```python
from build123d import *

# Parameters (mm, degrees)
F1_DEPTH = 12.7
F2_R     = 3.302
F3_DEPTH = 41.5002601562
F4_W     = 102.0685225816
F4_H     = 3.4845213629
F5_DEPTH = 25
F6_R     = 2


# Not quite as in the source:
# - ends of sketch curves that miss each other by under 0.0002 mm in the source are joined
# - the dataset's text gives a spline's control points without its knots; the knots are read off the source's solid


with BuildPart() as f1:
    # F0 (on Front) → F1 (new body)
    with BuildSketch(Plane.XZ):
        with BuildLine():
            Line((-8, 0), (0, 0))
            add(Edge.make_bspline(
                [(0, 0), (0, 16.0348825157), (7.430841215, 33.6514413357), (23.5, 33.5)],
                knots=[0, 0, 0, 0, 40.9206549312, 40.9206549312, 40.9206549312, 40.9206549312], degree=3))
            add(Edge.make_bspline(
                [(47, 0), (47, 16.0348825157), (39.569158785, 33.6514413357), (23.5, 33.5)],
                knots=[0, 0, 0, 0, 40.9206549312, 40.9206549312, 40.9206549312, 40.9206549312], degree=3))
            Line((47, 0), (55, 0))
            add(Edge.make_bspline(
                [(55, 0), (55, 2.3133051501), (54.8084752548, 5.6604865088), (54.3346414744, 8.9941225704), (54.1644875118, 10.0000161913)],
                knots=[0, 0, 0, 0, 0.125, 0.1792883855, 0.1792883855, 0.1792883855, 0.1792883855], degree=3))
            add(Edge.make_bspline(
                [(54.1644875118, 10.0000161913), (53.9428588652, 11.3102110198), (53.2041802455, 14.9199242801), (51.403557473, 20.6965522199), (48.312647429, 27.0635606249), (44.7757382973, 31.8590791464), (41.27501086, 35.2044913237), (38.3020149436, 37.39930019), (34.9881581098, 39.2038242784), (31.3670929719, 40.5407901401), (27.6491274865, 41.3170292606), (25.11417344, 41.4919330376), (23.9092731988, 41.5002601562)],
                knots=[0.1792883855, 0.1792883855, 0.1792883855, 0.1792883855, 0.25, 0.375, 0.5, 0.625, 0.6875, 0.75, 0.8125, 0.875, 0.9375, 0.9926226885, 0.9926226885, 0.9926226885, 0.9926226885], degree=3))
            Line((23.9092731988, 41.5002601562), (23.5, 41.5002601562))
            Line((23.5, 41.5002601562), (23.0907268012, 41.5002601562))
            add(Edge.make_bspline(
                [(-7.1644875118, 10.0000161913), (-6.9428588652, 11.3102110198), (-6.2041802455, 14.9199242801), (-4.403557473, 20.6965522199), (-1.312647429, 27.0635606249), (2.2242617027, 31.8590791464), (5.72498914, 35.2044913237), (8.6979850564, 37.39930019), (12.0118418902, 39.2038242784), (15.6329070281, 40.5407901401), (19.3508725135, 41.3170292606), (21.88582656, 41.4919330376), (23.0907268012, 41.5002601562)],
                knots=[0.1792883855, 0.1792883855, 0.1792883855, 0.1792883855, 0.25, 0.375, 0.5, 0.625, 0.6875, 0.75, 0.8125, 0.875, 0.9375, 0.9926226885, 0.9926226885, 0.9926226885, 0.9926226885], degree=3))
            add(Edge.make_bspline(
                [(-8, 0), (-8, 2.3133051501), (-7.8084752548, 5.6604865088), (-7.3346414744, 8.9941225704), (-7.1644875118, 10.0000161913)],
                knots=[0, 0, 0, 0, 0.125, 0.1792883855, 0.1792883855, 0.1792883855, 0.1792883855], degree=3))
        make_face()
        with BuildLine():
            Line((-23.5, 0), (-8, 0))
            add(Edge.make_bspline(
                [(-8, 0), (-8, 2.3133051501), (-7.8084752548, 5.6604865088), (-7.3346414744, 8.9941225704), (-7.1644875118, 10.0000161913)],
                knots=[0, 0, 0, 0, 0.125, 0.1792883855, 0.1792883855, 0.1792883855, 0.1792883855], degree=3))
            Line((-7.1644875118, 10.0000161913), (-23.5, 10))
            Line((-23.5, 10), (-23.5, 0))
        make_face()
        with BuildLine():
            Line((-23.5, 10), (-7.1643917939, 10))
            add(Edge.make_bspline(
                [(-7.1643917939, 10), (-6.9428588652, 11.3102110198), (-6.2041802455, 14.9199242801), (-4.403557473, 20.6965522199), (-1.312647429, 27.0635606249), (2.2242617027, 31.8590791464), (5.72498914, 35.2044913237), (8.6979850564, 37.39930019), (12.0118418902, 39.2038242784), (15.6329070281, 40.5407901401), (19.3508725135, 41.3170292606), (21.88582656, 41.4919330376), (23.0907268012, 41.5002601562)],
                knots=[0.1792883855, 0.1792883855, 0.1792883855, 0.1792883855, 0.25, 0.375, 0.5, 0.625, 0.6875, 0.75, 0.8125, 0.875, 0.9375, 0.9926226885, 0.9926226885, 0.9926226885, 0.9926226885], degree=3))
            Line((23.0907268012, 41.5002601562), (-23.5, 41.5002601562))
            Line((-23.5, 41.5002601562), (-23.5, 10))
        make_face()
        with BuildLine():
            add(Edge.make_bspline(
                [(55, 0), (55, 2.3133051501), (54.8084752548, 5.6604865088), (54.3346414744, 8.9941225704), (54.1644875118, 10.0000161913)],
                knots=[0, 0, 0, 0, 0.125, 0.1792883855, 0.1792883855, 0.1792883855, 0.1792883855], degree=3))
            Line((55, 0), (70.5, 0))
            Line((70.5, 0), (70.5, 10))
            Line((70.5, 10), (54.1644875118, 10.0000161913))
        make_face()
        with BuildLine():
            add(Edge.make_bspline(
                [(23.0907268012, 41.5002601562), (23.2269381476, 41.5012015188), (23.3633657228, 41.5012017791), (23.499999998, 41.5002598872)],
                knots=[0.9926226885, 0.9926226885, 0.9926226885, 0.9926226885, 0.9988541884, 0.9988541884, 0.9988541884, 0.9988541884], degree=3))
            Line((23.0907268012, 41.5002601562), (23.499999998, 41.5002598872))
        make_face()
        with BuildLine():
            add(Edge.make_bspline(
                [(54.1644875118, 10.0000161913), (53.9428588652, 11.3102110198), (53.2041802455, 14.9199242801), (51.403557473, 20.6965522199), (48.312647429, 27.0635606249), (44.7757382973, 31.8590791464), (41.27501086, 35.2044913237), (38.3020149436, 37.39930019), (34.9881581098, 39.2038242784), (31.3670929719, 40.5407901401), (27.6491274865, 41.3170292606), (25.11417344, 41.4919330376), (23.9092731988, 41.5002601562)],
                knots=[0.1792883855, 0.1792883855, 0.1792883855, 0.1792883855, 0.25, 0.375, 0.5, 0.625, 0.6875, 0.75, 0.8125, 0.875, 0.9375, 0.9926226885, 0.9926226885, 0.9926226885, 0.9926226885], degree=3))
            Line((54.1644875118, 10.0000161913), (70.5, 10))
            Line((70.5, 10), (70.5, 41.5002601562))
            Line((70.5, 41.5002601562), (23.9092731988, 41.5002601562))
        make_face()
        with BuildLine():
            add(Edge.make_bspline(
                [(23.9092731988, 41.5002601562), (23.7730618524, 41.5012015188), (23.6366342772, 41.5012017791), (23.500000002, 41.5002598872)],
                knots=[0.9926226885, 0.9926226885, 0.9926226885, 0.9926226885, 0.9988541884, 0.9988541884, 0.9988541884, 0.9988541884], degree=3))
            Line((23.500000002, 41.5002598872), (23.9092731988, 41.5002601562))
        make_face()
    extrude(amount=F1_DEPTH)

    # F2 (on face) → F3 (cut, through all)
    with BuildSketch(Plane.XY.offset(41.5002601562)):
        with Locations((-13.5000000019, -6.35)):
            Circle(F2_R)
        with Locations((60.4999999981, -6.35)):
            Circle(F2_R)
    extrude(amount=-F3_DEPTH, mode=Mode.SUBTRACT)

    # F4 (on Front) → F5 (cut)
    with BuildSketch(Plane.XZ):
        with Locations((22.9078933551, -0.7422606815)):
            Rectangle(F4_W, F4_H)
    extrude(amount=F5_DEPTH, mode=Mode.SUBTRACT)

    # F6
    f6_edges = [f1.edges().sort_by_distance(p)[0] for p in [
        (70.5, -6.35, 41.50026),
        (-23.5, -6.35, 41.50026),
    ]]
    fillet(f6_edges, radius=F6_R)


solid = f1.part
```
Input: part model. Units: mm. Frame: model coordinates. Round coordinates to 2 decimals unless told otherwise and drop trailing zeros. Loops run counter-clockwise (first coordinate to the right, second up) from the corner with the lowest first, then second, coordinate; pieces in that order, holes last. Notation, with made-up numbers: (56.5, -29) -> (87.5, -29) arc R34 ccw to (87.5, 7) -> close; hole circle Ø6 at (-36, 73.25). An arc over 180 degrees is marked (long way). Use one line per item in the form item = value. Start each with the question number.
Item 1: Section query A-A on x = -13.5. Return the cut outline in (y, z), then the cut area to 3 significant figures.
Item 2: Material intervals for L1, parallel to Y at x = 60.5, z = 10; L2, parallel to Y at x = 60, z = 19; L3, parallel to X at y = -3.5, z = 28.5, sorted ascending. Write a range as from..to.
Item 3: Mould query, pull axis X, two halves, no side actions, for faces 1 (the face through (-22.93, -6.44, 40.9)), 2 (the face through (-16.8, -6.2, 21.5)), 3 (the face through (1, -6, 41.5)). Classes: pulls with the +X half, pulls with the -X half, needs draft (parallel to the pull), parting line crosses it, or undercut.
Item 4: Contact query for flat-ended pins moving along their axis: pin 1 Ø3 at (x, y) = (36.5, -4) entering from -Z; pin 2 Ø5.5 at (x, y) = (-13.5, -6.35) entering from +Z. Output: stop coordinate, or through.
Item 5: Section query B-B on z = 20. Count the separate pieces of the cut face and the enclosed holes in it, then the cut area to 3 significant figures.
Ans:
q1.outline = (-12.7, 1) -> (-9.65, 1) -> (-9.65, 41.5) -> (-12.7, 41.5) -> close; (-3.05, 1) -> (0, 1) -> (0, 41.5) -> (-3.05, 41.5) -> close
q1.area = 247 mm^2
q2.L1 = -12.7..-9.65, -3.05..0
q2.L2 = -12.7..-9.61, -3.09..0
q2.L3 = -23.5..-15.17, -11.83..10.33, 36.67..58.83, 62.17..70.5
q3.face_1 = pulls with the -X half
q3.face_2 = undercut
q3.face_3 = needs draft
q4.pin_1 = 27.19
q4.pin_2 = through
q5.separate_pieces = 2
q5.enclosed_holes = 2
q5.area = 635 mm^2
